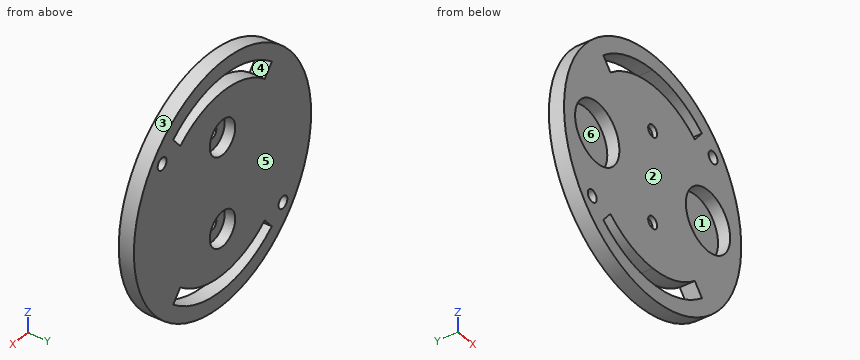
Autodesk Inventor part; units mm, degrees
ref_plane "Work Plane1" through (0, 0, -32.5) normal (1, 0, 0) x (0, 0, -1)
ref_plane "YZ Plane" through (0, 0, 0) normal (1, 0, 0) x (0, 1, 0)
ref_plane "XZ Plane" through (0, 0, 0) normal (0, 1, 0) x (-1, 0, 0)
sketch "Sketch1" plane through (0, 0, 0) normal (0, 1, 0) x (-1, 0, 0)
  circle A0 centre (0, 0) radius 40
  dimension "d0" = 80
sketch "Sketch1 outline for Extrusion1" plane through (0, 0, 0) normal (0, 1, 0) x (-1, 0, 0)
  circle A0 centre (0, 0) radius 40
extrude "Extrusion1" add sketch "Sketch1 outline for Extrusion1" along normal blind 5
sketch "Sketch6" plane through (0, 0, 0) normal (0, -1, 0) x (1, 0, 0)
  line L0 (0, 0) -> (25, 0)
  circle A0 centre (25, 0) radius 10
  line L1 (0, 0) -> (-25, 0)
  line L2 (0, 0) -> (25, 0) construction
  circle A1 centre (-25, 0) radius 10
  dimension "d19" = 25
  dimension "d20" = 20
  dimension "d46" = 25
  dimension "d47" = 180
  dimension "d48" = 20
sketch "Sketch6 outline for Extrusion5" plane through (0, 0, 0) normal (0, -1, 0) x (1, 0, 0)
  circle A0 centre (25, 0) radius 10
  circle A1 centre (-25, 0) radius 10
extrude "Extrusion5" cut sketch "Sketch6 outline for Extrusion5" against normal blind 4
sketch "Sketch8" plane through (0, 0, 0) normal (0, -1, 0) x (1, 0, 0)
  circle A0 centre (0, 0) radius 40
  line L0 (21.650635, 27.5) -> (26.777009, 27.5) construction
  line L1 (0, 40) -> (0, 35)
  circle A1 centre (0, 0) radius 35
  line L2 (0, 35) -> (0, 30)
  circle A2 centre (0, 0) radius 30
  line L3 (0, 30) -> (26.457513, 30)
  line L4 (18.027756, 30) -> (15.52731, 25.669099)
  line L5 (18.027756, 30) -> (23.02865, 30) construction
  line L6 (-40, 0) -> (40, 0)
  line L7 (0, -30) -> (0, -40)
  line L8 (0, 30) -> (0, 27)
  line L9 (0, 27) -> (29.512709, 27)
  line L10 (22.271057, 27) -> (27.352779, 27) construction
  line L11 (22.271057, 27) -> (19.056987, 23.169619)
  line L12 (22.271057, 27) -> (27.271264, 27) construction
  line L13 (22.271057, -27) -> (19.056987, -23.169619)
  point P0 (0, -35)
  dimension "d53" = 5
  dimension "d54" = 5
  dimension "d55" = 120
  dimension "d58" = 3
  dimension "d60" = 130
sketch "Sketch8 outline for Extrusion7" plane through (0, 0, 0) normal (0, -1, 0) x (1, 0, 0)
  line L0 (22.271057, -27) -> (19.056987, -23.169619)
  arc A0 (0, -35) -> (22.271057, -27) centre (0, 0) ccw
  line L1 (0, -30) -> (0, -35)
  arc A1 (19.056987, -23.169619) -> (0, -30) centre (0, 0) cw
  line L2 (19.056987, 23.169619) -> (22.271057, 27)
  arc A2 (0, 30) -> (19.056987, 23.169619) centre (0, 0) cw
  line L3 (0, 35) -> (0, 30)
  arc A3 (22.271057, 27) -> (0, 35) centre (0, 0) ccw
extrude "Extrusion7" cut sketch "Sketch8 outline for Extrusion7" against normal up to surface (5 mm away)
ref_plane "Work Plane1" through (0, 0, -32.5) normal (1, 0, 0) x (0, 0, -1)
mirror "Mirror1" about plane through (0, 0, -32.5) normal (1, 0, 0) of "Extrusion7"
sketch "Sketch9" plane through (0, 5, 0) normal (0, 1, 0) x (1, 0, 0)
  circle A0 centre (25, 0) radius 10
  circle A1 centre (-25, 0) radius 10
  arc A2 (-19.056987, -23.169619) -> (19.056987, -23.169619) centre (0, 0) ccw
  line L0 (0, 0) -> (0, -30)
  line L1 (0, 0) -> (0, 30)
  arc A3 (19.056987, 23.169619) -> (-19.056987, 23.169619) centre (0, 0) ccw
  line L2 (0, 0) -> (0, -15)
  circle A4 centre (0, -15) radius 5.75
  line L3 (0, 0) -> (0, 15)
  circle A5 centre (0, 15) radius 5.75
  dimension "d61" = 15
  dimension "d62" = 11.5
  dimension "d63" = 15
  dimension "d64" = 11.5
sketch "Sketch9 outline for Extrusion8" plane through (0, 5, 0) normal (0, 1, 0) x (1, 0, 0)
  circle A0 centre (0, 15) radius 5.75
  circle A1 centre (0, -15) radius 5.75
extrude "Extrusion8" cut sketch "Sketch9 outline for Extrusion8" against normal blind 3.5
sketch "Sketch10" plane through (0, 1.5, 15) normal (0, 1, 0) x (1, 0, 0)
  circle A0 centre (0, 30) radius 5.75
  circle A1 centre (0, 30) radius 2
  circle A2 centre (0, 0) radius 5.75
  circle A3 centre (0, 0) radius 2
  point P0 (0, 15)
  dimension "d68" = 4
  dimension "d69" = 4
sketch "Sketch10 outline for Extrusion9" plane through (0, 1.5, 15) normal (0, 1, 0) x (1, 0, 0)
  circle A0 centre (0, 0) radius 2
  circle A1 centre (0, 30) radius 2
extrude "Extrusion9" cut sketch "Sketch10 outline for Extrusion9" against normal up to surface (1.5 mm away)
sketch "Sketch11" plane through (0, 0, 0) normal (0, -1, 0) x (1, 0, 0)
  line L0 (22.271057, 27) -> (19.056987, 23.169619)
  line L1 (22.271057, 27) -> (22.271057, 22)
  line L2 (22.271057, 22) -> (27.271057, 22)
  circle A0 centre (27.271057, 22) radius 2
  arc A1 (-22.271057, -27) -> (22.271057, -27) centre (0, 0) ccw
  line L3 (-22.271057, -27) -> (-22.271057, -22)
  line L4 (-22.271057, -22) -> (-27.271057, -22)
  circle A2 centre (-27.271057, -22) radius 2
  dimension "d72" = 5
  dimension "d73" = 5
  dimension "d74" = 4
  dimension "d75" = 5
  dimension "d76" = 5
  dimension "d77" = 4
sketch "Sketch11 outline for Extrusion10" plane through (0, 0, 0) normal (0, -1, 0) x (1, 0, 0)
  circle A0 centre (27.271057, 22) radius 2
  circle A1 centre (-27.271057, -22) radius 2
extrude "Extrusion10" cut sketch "Sketch11 outline for Extrusion10" against normal up to surface (5 mm away)
properties part number "Wrist_Coupling"
The model under review builds one solid part; all positions refer to its coordinate system, in mm. Face numbers are marked on the shaded views. A direction names the side the tool comes from. Round coordinates to 2 decimals unless told otherwise and drop trailing zeros. Write each loop counter-clockwise with the first axis right and the second up, starting at its lowest first coordinate (ties: lowest second). Pieces come first, ordered by that corner, then holes. Notation, with made-up numbers: (22, -35.5) -> (70, -35.5) arc R17 cw to (70, -12.5) -> close; hole circle Ø11 at (43.5, -16). An arc over 180 degrees is marked (long way). Use CSV: the item, a comma, the result in double quotes.
Q1. Consider section C-C (z = 22). Give the boundary of the cut face in (x, y).
Checks:
outline,"(-33.41, 0) -> (25.27, 0) -> (25.27, 5) -> (-33.41, 5) -> close; (29.27, 0) -> (33.41, 0) -> (33.41, 5) -> (29.27, 5) -> close"
Q2. Consider section D-D (z = 0). Give the boundary of the cut face in (x, y).
Checks:
outline,"(-40, 0) -> (-35, 0) -> (-35, 4) -> (-15, 4) -> (-15, 0) -> (15, 0) -> (15, 4) -> (35, 4) -> (35, 0) -> (40, 0) -> (40, 5) -> (-40, 5) -> close"
Q3. To check wall thickness, follow probe 1 along Z at (x, y) = (0, 2.3); probe 2 along Z at (x, y) = (-22, 1.6); probe 3 along Z at (x, y) = (16, 3.5). State the ranges of each line that lie inside material, in increasing order. Write a range as [from, to].
Checks:
probe 1,"[-40, -35], [-30, -20.75], [-9.25, 9.25], [20.75, 30], [35, 40]"
probe 2,"[-33.41, -27.22], [-26.68, -9.54], [9.54, 26.68], [27.22, 33.41]"
probe 3,"[-36.66, -31.13], [-25.38, -4.36], [4.36, 25.38], [31.13, 36.66]"
Q4. For the marked faces 5 and 6, list the 3-axis set-ups (+Z, -Z, +X, -X, +Y, -Y) from which the entire face can be reached by the end or side of a thin tool; tool diameter is ignored.
Checks:
face 5,"+Z, -Z, +X, -X, +Y"
face 6,"-Y"
Q5. Mouldability with a two-part tool opening along Z and no side actions: class the marked faces 1, 2, 3 and 4 as released by +Z, released by -Z, zero draft, split by the parting line, or undercut.
Checks:
face 1,"undercut"
face 2,"zero draft"
face 3,"split by the parting line"
face 4,"undercut"
Q6. For pin 1 Ø6 at (x, z) = (25.5, 2) entering from -Y; pin 2 Ø2 at (y, z) = (2.5, 25) entering from +X; pin 3 Ø1 at (y, z) = (2.5, 29) entering from -X, all flat-tipped, find the tip position at first contact; note any pin that passes through.
Checks:
pin 1,"y = 4"
pin 2,"x = 32"
pin 3,"x = -28.07"
